Geometry check sheet. Reference: drawing and pictorial views, mm from the part's lowest x, y, z. A direction names the side the tool comes from. Round coordinates to 2 decimals unless told otherwise and drop trailing zeros. Write each loop counter-clockwise with the first axis right and the second up, starting at its lowest first coordinate (ties: lowest second). Pieces come first, ordered by that corner, then holes. Notation, with made-up numbers: (75, -2.75) -> (95, -2.75) arc R22 cw to (95, 31.25) -> close; hole circle Ø2 at (3, -22.75). An arc over 180 degrees is marked (long way). Answer as a JSON object with one key per item and string values. Group by question number.
(1) Set-up check for the marked faces 1, 2 and 3: record each of +Z, -Z, +X, -X, +Y, -Y from which the full face is reachable in a straight line by a thin tool's end or side.
(2) Scan lines: L1, parallel to Z at x = 25.5, y = 13.75 (1 decimal); L2, parallel to X at y = 7, z = 45; L3, parallel to Z at x = 26, y = 9.5. Record each from-to range of solid material in increasing order. Write a range as from..to.
(3) Sectioned sample at B-B on x = 26. Record the cut outline in (y, z), and give its area (3 significant figures).
(4) Sectioned sample at A-A on z = 26. Record the cut outline in (x, y), and give its area (3 significant figures).
(5) Sectioned sample at D-D on z = 47. Record the cut outline in (x, y), and give its area (3 significant figures).
(6) Sectioned sample at C-C on y = 1. Record the cut outline in (x, z), and give its area (3 significant figures).
(7) Draft check along Z on the marked faces 4, 5 and 6. Enter one of: released by +Z, released by -Z, zero draft, split by the parting line, or undercut.
(8) Gauge pin test, flat ends, axial feed: pin 1 Ø9.5 at (x, z) = (6, 29.5) entering from +Y; pin 2 Ø4.5 at (x, z) = (45, 20.5) entering from -Y; pin 3 Ø6 at (x, y) = (18.5, 12) entering from -Z; pin 4 Ø1.5 at (y, z) = (5.5, 38) entering from +X. Record the tip position at first contact, or that the pin passes through.
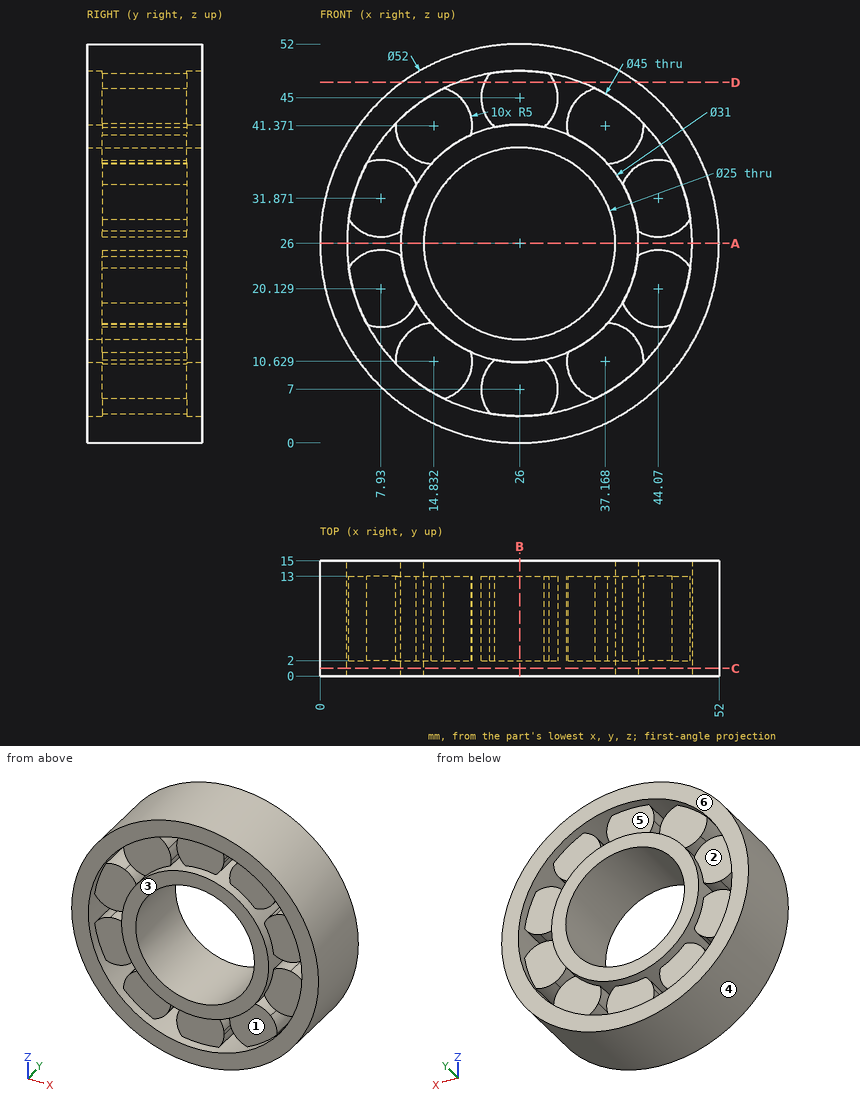
Computed values:
{
 "1": {"face 1": "-Y", "face 2": "+Y", "face 3": "+Z, -Z, +X, -X, -Y"},
 "2": {"L1": "0..3.5, 10.5..13.5, 38.5..41.5, 48.5..52", "L2": "8.25..18.27, 21..31, 33.73..43.75", "L3": "0..13.5, 38.5..52"},
 "3": {"outline": "(0, 0) -> (15, 0) -> (15, 3.5) -> (13, 3.5) -> (13, 10.5) -> (15, 10.5) -> (15, 13.5) -> (0, 13.5) -> (0, 10.5) -> (2, 10.5) -> (2, 3.5) -> (0, 3.5) -> close; (0, 38.5) -> (15, 38.5) -> (15, 41.5) -> (13, 41.5) -> (13, 48.5) -> (15, 48.5) -> (15, 52) -> (0, 52) -> (0, 48.5) -> (2, 48.5) -> (2, 41.5) -> (0, 41.5) -> close", "area": "349 mm2"},
 "4": {"outline": "(0, 0) -> (3.5, 0) -> (3.5, 15) -> (0, 15) -> close; (10.5, 0) -> (13.5, 0) -> (13.5, 15) -> (10.5, 15) -> close; (38.5, 0) -> (41.5, 0) -> (41.5, 15) -> (38.5, 15) -> close; (48.5, 0) -> (52, 0) -> (52, 15) -> (48.5, 15) -> close", "area": "195 mm2"},
 "5": {"outline": "(10.67, 0) -> (17.92, 0) -> (17.92, 15) -> (10.67, 15) -> close; (21.42, 2) -> (30.58, 2) -> (30.58, 13) -> (21.42, 13) -> close; (34.08, 0) -> (41.33, 0) -> (41.33, 15) -> (34.08, 15) -> close", "area": "318 mm2"},
 "6": {"outline": "circle Ø52 at (26, 26); circle Ø31 at (26, 26); hole circle Ø45 at (26, 26); hole circle Ø25 at (26, 26)", "area": "797 mm2"},
 "7": {"face 4": "split by the parting line", "face 5": "undercut", "face 6": "zero draft"},
 "8": {"pin 1": "y = 15", "pin 2": "y = 2", "pin 3": "z = 0.39", "pin 4": "x = 49.44"}
}
